The drawing under review shows one solid part. Ordinate dimensions are in mm from its lowest x, y, z. Round coordinates to 2 decimals unless told otherwise and drop trailing zeros. Write each loop counter-clockwise with the first axis right and the second up, starting at its lowest first coordinate (ties: lowest second). Pieces come first, ordered by that corner, then holes. Notation, with made-up numbers: (38, -35) -> (85, -35) arc R24 cw to (85, 0) -> close; hole circle Ø1 at (-28.5, -8.5). An arc over 180 degrees is marked (long way). Use CSV: the item, a comma, the result in double quotes. Start each with the question number.
1) Take a section at D-D, the plane y = 3.5. Give the boundary of the cut face in (x, z).
2) Take a section at A-A, the plane z = 4. Give the boundary of the cut face in (x, y).
3) Wall thickness on probe 1 along Z at (x, y) = (11.5, 7.5); probe 2 along X at (y, z) = (17.25, 4); probe 3 along Z at (x, y) = (9.75, 8.75): over which ranges is each line inside the solid? List them lowest first. Write a range as [from, to].
4) For pin 1 Ø8 at (x, y) = (9, 18.5) entering from -Z; pin 2 Ø5.5 at (x, z) = (9.47, 4) entering from +Y, all flat-tipped, find the tip position at first contact; note any pin that passes through.
5) Take a section at C-C, the plane x = 7.5. Give the boundary of the cut face in (y, z), then the cut area to 3 significant figures.
6) Mouldability with a two-part tool opening along Z and no side actions: class the marked faces 1, 2 and 3 as released by +Z, released by -Z, zero draft, split by the parting line, or undercut.
7) Take a section at B-B, the plane y = 6.5. Give the boundary of the cut face in (x, z), then the cut area to 3 significant figures.
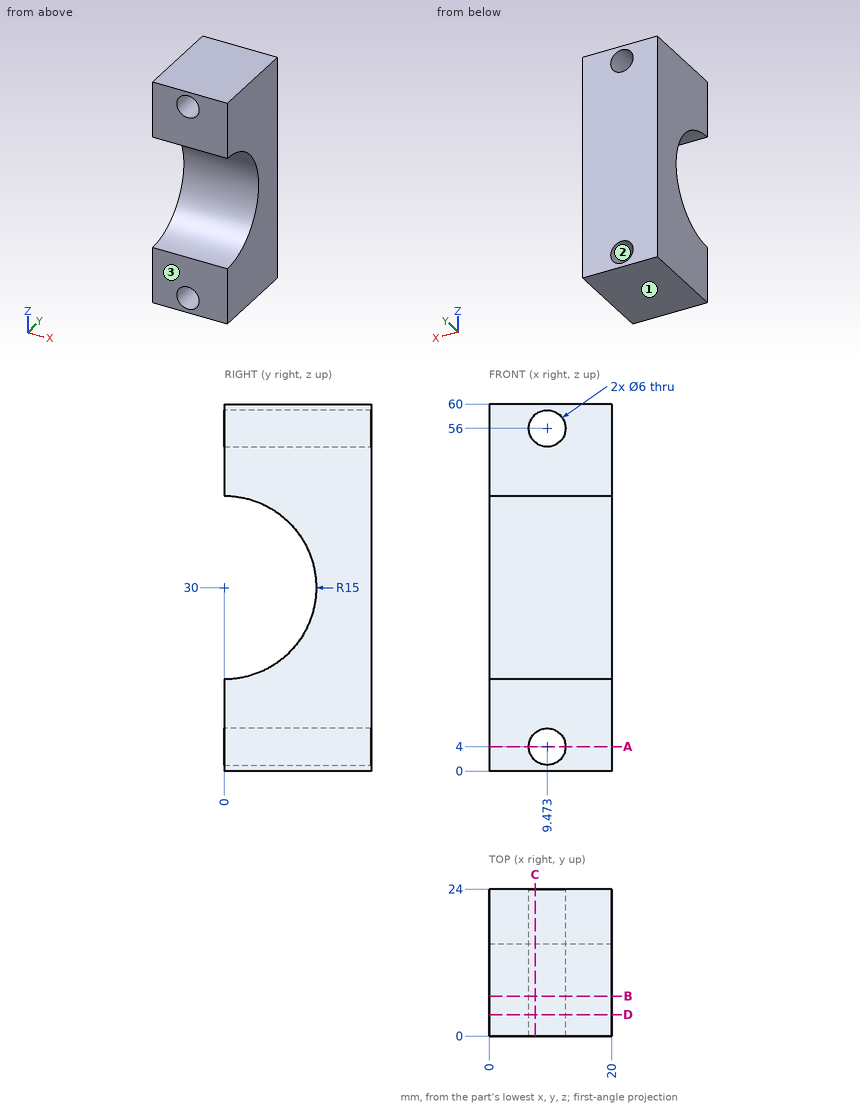
Values found:
1,outline,"(0, 0) -> (20, 0) -> (20, 15.41) -> (0, 15.41) -> close; (0, 44.59) -> (20, 44.59) -> (20, 60) -> (0, 60) -> close; hole circle Ø6 at (9.47, 4); hole circle Ø6 at (9.47, 56)"
2,outline,"(0, 0) -> (6.47, 0) -> (6.47, 24) -> (0, 24) -> close; (12.47, 0) -> (20, 0) -> (20, 24) -> (12.47, 24) -> close"
3,probe 1,"[0, 1.79], [6.21, 17.01], [42.99, 53.79], [58.21, 60]"
3,probe 2,"[0, 6.47], [12.47, 20]"
3,probe 3,"[0, 1.01], [6.99, 17.82], [42.18, 53.01], [58.99, 60]"
4,pin 1,"z = 0"
4,pin 2,"through"
5,outline,"(0, 0) -> (24, 0) -> (24, 1.74) -> (0, 1.74) -> close; (0, 6.26) -> (24, 6.26) -> (24, 53.74) -> (0, 53.74) -> (0, 45) arc R15 cw to (0, 15) -> close; (0, 58.26) -> (24, 58.26) -> (24, 60) -> (0, 60) -> close"
5,area,"870 mm²"
6,face 1,"released by -Z"
6,face 2,"undercut"
6,face 3,"zero draft"
7,outline,"(0, 0) -> (20, 0) -> (20, 16.48) -> (0, 16.48) -> close; (0, 43.52) -> (20, 43.52) -> (20, 60) -> (0, 60) -> close; hole circle Ø6 at (9.47, 4); hole circle Ø6 at (9.47, 56)"
7,area,"603 mm²"
